from build123d import *

# Parameters (mm, degrees)
CROQUIS3_W              = 92
CROQUIS3_H              = 482
CROQUIS3_R              = 2.5
CROQUIS3_R_2            = 2
CROQUIS3_R_3            = 5
CROQUIS3_R_4            = 1.5
CROQUIS3_R_5            = 6
SALIENTE_EXTRUIR1_DEPTH = 4


with BuildPart() as part:
    # Croquis3 → Saliente-Extruir1 (new body)
    with BuildSketch(Plane.ZY.offset(90.501614904)):
        with Locations((-42, 944.628389678)):
            Rectangle(CROQUIS3_W, CROQUIS3_H)
        with Locations((-80.223774801, 783.628389678)):
            Circle(CROQUIS3_R, mode=Mode.SUBTRACT)
        with Locations((-67.682201304, 768.118311041)):
            Circle(CROQUIS3_R_2, mode=Mode.SUBTRACT)
        with Locations((-67.682201304, 800.118311041)):
            Circle(CROQUIS3_R_2, mode=Mode.SUBTRACT)
        with Locations((-35.682201304, 800.118311041)):
            Circle(CROQUIS3_R_2, mode=Mode.SUBTRACT)
        with Locations((-35.682201304, 768.118311041)):
            Circle(CROQUIS3_R_2, mode=Mode.SUBTRACT)
        with Locations((-22.223774801, 783.628389678)):
            Circle(CROQUIS3_R, mode=Mode.SUBTRACT)
        with Locations((-67.682201304, 860.118311041)):
            Circle(CROQUIS3_R_2, mode=Mode.SUBTRACT)
        with Locations((-67.682201304, 892.118311041)):
            Circle(CROQUIS3_R_2, mode=Mode.SUBTRACT)
        with Locations((-35.682201304, 892.118311041)):
            Circle(CROQUIS3_R_2, mode=Mode.SUBTRACT)
        with Locations((-35.682201304, 860.118311041)):
            Circle(CROQUIS3_R_2, mode=Mode.SUBTRACT)
        with Locations((-22.223774801, 875.628389678)):
            Circle(CROQUIS3_R, mode=Mode.SUBTRACT)
        with Locations((-51.223774801, 907.728389678)):
            Circle(CROQUIS3_R_3, mode=Mode.SUBTRACT)
        with Locations((-51.223774801, 928.11276849)):
            Circle(CROQUIS3_R_4, mode=Mode.SUBTRACT)
        with Locations((-44.223774801, 944.628389678)):
            Circle(CROQUIS3_R_5, mode=Mode.SUBTRACT)
        with Locations((-37.360604168, 936.116673787)):
            Circle(CROQUIS3_R_4, mode=Mode.SUBTRACT)
        with Locations((-37.360604168, 952.124484381)):
            Circle(CROQUIS3_R_4, mode=Mode.SUBTRACT)
        with Locations((-51.223774801, 960.128389678)):
            Circle(CROQUIS3_R_4, mode=Mode.SUBTRACT)
        with Locations((-65.086945434, 952.124484381)):
            Circle(CROQUIS3_R_4, mode=Mode.SUBTRACT)
        with Locations((-65.086945434, 936.116673787)):
            Circle(CROQUIS3_R_4, mode=Mode.SUBTRACT)
        with Locations((-80.223774801, 1013.628389678)):
            Circle(CROQUIS3_R, mode=Mode.SUBTRACT)
        with Locations((-22.223774801, 1013.628389678)):
            Circle(CROQUIS3_R, mode=Mode.SUBTRACT)
        with Locations((-22.223774801, 1105.628389678)):
            Circle(CROQUIS3_R, mode=Mode.SUBTRACT)
        with Locations((-80.223774801, 1105.628389678)):
            Circle(CROQUIS3_R, mode=Mode.SUBTRACT)
        with Locations((-80.223774801, 875.628389678)):
            Circle(CROQUIS3_R, mode=Mode.SUBTRACT)
        with BuildLine():
            Line((-67.682201304, 795.421766265), (-67.682201304, 772.814855817))
            ThreePointArc((-67.682201304, 772.814855817), (-71.272201304, 784.118311041), (-67.682201304, 795.421766265))
        make_face(mode=Mode.SUBTRACT)
        Polygon((-59.682201304, 802.000371885), (-59.682201304, 766.236250198), (-63.865689893, 768.777818683), (-63.682201304, 799.602758077), align=None, mode=Mode.SUBTRACT)
        Polygon((-55.682201304, 803.29559187), (-55.682201304, 764.941030212), (-51.682201304, 764.528311041), (-51.682201304, 803.708311041), align=None, mode=Mode.SUBTRACT)
        Polygon((-47.682201304, 803.29559187), (-47.682201304, 764.941030212), (-43.682201304, 766.236250198), (-43.682201304, 802.000371885), align=None, mode=Mode.SUBTRACT)
        Polygon((-39.682201304, 799.602758077), (-39.498712715, 768.777818683), (-35.682201304, 772.814855817), (-35.682201304, 795.421766265), align=None, mode=Mode.SUBTRACT)
        Polygon((-35.682201304, 887.421766265), (-39.498712715, 891.4588034), (-39.682201304, 860.633864006), (-35.682201304, 864.814855817), align=None, mode=Mode.SUBTRACT)
        Polygon((-43.682201304, 894.000371885), (-47.682201304, 895.29559187), (-47.682201304, 856.941030212), (-43.682201304, 858.236250198), align=None, mode=Mode.SUBTRACT)
        Polygon((-51.682201304, 895.708311041), (-55.682201304, 895.29559187), (-55.682201304, 856.941030212), (-51.682201304, 856.528311041), align=None, mode=Mode.SUBTRACT)
        Polygon((-59.682201304, 894.000371885), (-63.865689893, 891.4588034), (-63.682201304, 860.633864006), (-59.682201304, 858.236250198), align=None, mode=Mode.SUBTRACT)
    extrude(amount=SALIENTE_EXTRUIR1_DEPTH)


solid = part.part
Check sheet for the modelled part. Datum: model origin and axes. Units: mm. Give positions to 0.01 mm unless a question says otherwise; leave off trailing zeros. One line per item, written item: value. Start each with the question number.
Item 1: Section check A-A on x = -91.6. State how many separate pieces and enclosed holes the cut face has, then the cut area to 3 significant figures.
Item 2: Gauge pin test, flat ends, axial feed: pin 1 (4 mm diameter, centred on y = 1105.63, z = -80.22, fed in from -X); pin 2 (8 mm diameter, centred on y = 783.63, z = -22.22, fed in from -X). Record the tip position at first contact, or that the pin passes through.
Item 3: Material ranges on probe 1 along Y at (x, z) = (-91.65, -80); probe 2 along Y at (x, z) = (-92.9, -35.5); probe 3 along Y at (x, z) = (-93.55, -49.5), recorded low to high. Write a range as from..to.
Item 4: Draft check along Z on faces 1 (the flat face through (-90.502, 948, -32)), 2 (the cylindrical face through (-92.5, 903.3, -48.9)). Enter one of: +Z half, -Z half, draft (parallel to the pull), parting line (faces both ways), or undercut.
Results list:
1. separate pieces: 1
1. enclosed holes: 33
1. area: 42,700 mm²
2. pin 1: through
2. pin 2: x = -94.5
3. probe 1: 703.63..781.14, 786.12..873.14, 878.12..1011.14, 1016.12..1103.14, 1108.12..1185.63
3. probe 2: 703.63..766.13, 770.11..798.13, 802.11..858.13, 862.11..890.13, 894.11..1185.63
3. probe 3: 703.63..903.03, 912.42..941.77, 947.49..1185.63
4. face 1: draft
4. face 2: undercut
